Solid Edge part; units mm, degrees
sketch "Sketch1" plane through (0, 0, 0) normal (0, 0, 1) x (1, 0, 0)
  line L0 (-10, -5.25) -> (10, -5.25)
  line L1 (10, -5.25) -> (10, 5.25)
  line L2 (10, 5.25) -> (-10, 5.25)
  line L3 (-10, 5.25) -> (-10, -5.25)
  dimension "D1" = 10
extrude "Protrusion1" add sketch "Sketch1" along normal blind 6.5
sketch "Sketch2" plane through (0, 0, 6.5) normal (0, 0, 1) x (1, 0, 0)
  circle A0 centre (5.85, -2.25) radius 1
  circle A1 centre (-5.85, -2.25) radius 1
  dimension "D1" = 5.85
extrude "ExtrudedCutout_1" cut sketch "Sketch2" against normal blind 40.1808
sketch "Sketch3" plane through (0, 5.25, 3.25) normal (0, 1, 0) x (1, 0, 0)
  line L0 (-8.9539, 3.25) -> (-8.9539, -3.25)
  line L1 (-8.9539, -3.25) -> (8.9539, -3.25)
  line L2 (8.9539, -3.25) -> (8.9539, 3.25)
  line L3 (8.9539, 3.25) -> (-8.9539, 3.25)
extrude "ExtrudedProtrusion_2" add sketch "Sketch3" along normal blind 0.85
Geometry check sheet. Reference: the model listing, model coordinates, mm. A direction names the side the tool comes from. Give positions to 0.01 mm unless a question says otherwise; leave off trailing zeros. Order: outer loops, then holes, each group sorted by start corner. A loop starts at its lowest first (then second) coordinate and runs counter-clockwise, first axis right, second up. Notation, with made-up numbers: (38, -12.5) - (80, -12.5) arc R37 ccw to (80, 24.5) - close; hole circle Ø4 at (72, 64.5). An arc over 180 degrees is marked (long way). Use one line per item in the form item = value.
1) Sectioned sample at B-B (z = 1.5). Record the boundary of the cut face in (x, y), and give its area (3 significant figures).
Working result:
outline = (-10, -5.25) - (10, -5.25) - (10, 5.25) - (8.95, 5.25) - (8.95, 6.1) - (-8.95, 6.1) - (-8.95, 5.25) - (-10, 5.25) - close; hole circle Ø2 at (-5.85, -2.25); hole circle Ø2 at (5.85, -2.25)
area = 219 mm^2
2) Sectioned sample at A-A (y = -2.25). Record the boundary of the cut face in (x, z).
Working result:
outline = (-10, 0) - (-6.85, 0) - (-6.85, 6.5) - (-10, 6.5) - close; (-4.85, 0) - (4.85, 0) - (4.85, 6.5) - (-4.85, 6.5) - close; (6.85, 0) - (10, 0) - (10, 6.5) - (6.85, 6.5) - close
3) Depth check by flat-ended pin: pin 1 Ø0.5 at (x, z) = (-9.5, 3) entering from +Y; pin 2 Ø0.7 at (y, z) = (6, 2) entering from -X; pin 3 Ø2.5 at (x, y) = (-5.85, -2.25) entering from +Z; pin 4 Ø0.9 at (y, z) = (6, 4) entering from +X. Enter the tip coordinate at first touch or a pass-through.
Working result:
pin_1 = 5.25
pin_2 = -8.95
pin_3 = 6.5
pin_4 = 8.95
4) Draft check along Y on faces 1 (the face through (6.31, -3.14, 3.3)), 2 (the face through (8.954, 5.7, 3.3)), 3 (the face through (-9.5, 5.25, 3.2)). Enter one of: released by +Y, released by -Y, zero draft, split by the parting line, or undercut.
Working result:
face_1 = undercut
face_2 = zero draft
face_3 = released by +Y
5) Access from +Z, -Z, +X, -X, +Y, -Y to the whole of each face (thin tool, end or side, straight path). Record for faces 4 (the face through (0, 1, 0)), 5 (the face through (9.5, 5.25, 3.2)), 6 (the face through (-8.954, 5.7, 3.2)).
Working result:
face_4 = -Z, +X, -X, +Y, -Y
face_5 = +Z, -Z, +X, +Y
face_6 = +Z, -Z, -X, +Y
6) Sectioned sample at C-C (x = 5.85). Record the boundary of the cut face in (y, z).
Working result:
outline = (-5.25, 0) - (-3.25, 0) - (-3.25, 6.5) - (-5.25, 6.5) - close; (-1.25, 0) - (6.1, 0) - (6.1, 6.5) - (-1.25, 6.5) - close
7) Material ranges on probe 1 along X at (y, z) = (-3, 1); probe 2 along Y at (x, z) = (5.85, 1.5); probe 3 along X at (y, z) = (-2.75, 6.25), recorded low to high. Write a range as from..to.
Working result:
probe_1 = -10..-6.51, -5.19..5.19, 6.51..10
probe_2 = -5.25..-3.25, -1.25..6.1
probe_3 = -10..-6.72, -4.98..4.98, 6.72..10
